Verification items for this drawing (mm, ordinates from the low corner). Give positions to 0.01 mm unless a question says otherwise; leave off trailing zeros. Loops run counter-clockwise (first coordinate to the right, second up) from the corner with the lowest first, then second, coordinate; pieces in that order, holes last. Notation, with made-up numbers: M 44.25,24.25 L 97.25,24.25 A31 ccw 97.25,54.25 Z; hole C 18.25,73.25 d8. An arc over 180 degrees is marked long. Use one line per item in the form item = value.
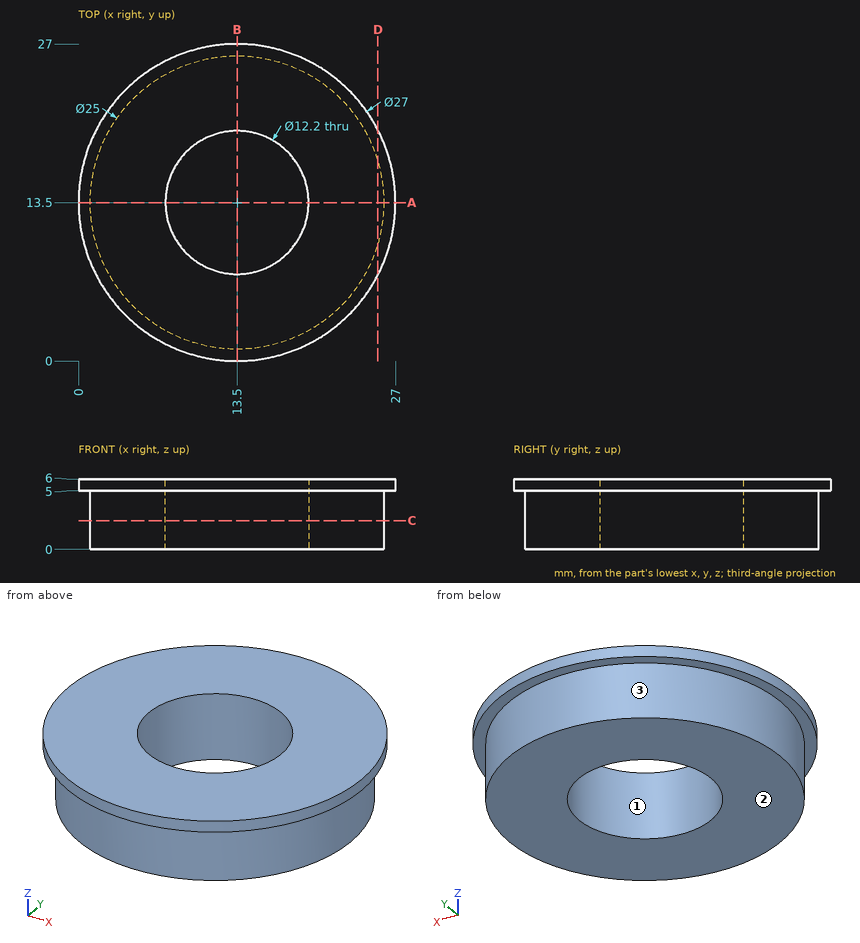
1) Depth check by flat-ended pin: pin 1 Ø1 at (x, z) = (17.5, 3.5) entering from -Y; pin 2 Ø4 at (x, y) = (20.5, 7) entering from -Z; pin 3 Ø1.5 at (x, z) = (21, 4) entering from -Y. Enter the tip coordinate at first touch or a pass-through.
Evaluation:
pin_1 = 1.5
pin_2 = 0
pin_3 = 2.98
2) Section check D-D (x = 25.5). Record the cut outline in (y, z), then the cut area to 3 significant figures.
Evaluation:
outline = M 7.32,5 L 10,5 L 10,0 L 17,0 L 17,5 L 19.68,5 L 19.68,6 L 7.32,6 Z
area = 47.4 mm^2
3) Section check C-C (z = 2.45). Record the cut outline in (x, y), then the cut area to 3 significant figures.
Evaluation:
outline = C 13.5,13.5 d25; hole C 13.5,13.5 d12.2
area = 374 mm^2
4) Section check A-A (y = 13.5). Record the cut outline in (x, z).
Evaluation:
outline = M 0,5 L 1,5 L 1,0 L 7.4,0 L 7.4,6 L 0,6 Z; M 19.6,0 L 26,0 L 26,5 L 27,5 L 27,6 L 19.6,6 Z
5) Release check for a two-part mould opening along X. For the marked faces 1, 2 and 3 record: pulls with the +X half, pulls with the -X half, needs draft (parallel to the pull), parting line crosses it, or undercut.
Evaluation:
face_1 = undercut
face_2 = needs draft
face_3 = parting line crosses it
6) Scan lines: line 1 (Y direction, x = 13.5, z = 4.1); line 2 (Z direction, x = 25.75, y = 9.5); line 3 (Y direction, x = 18.5, z = 3.9). Record each from-to range of solid material in increasing order.
Evaluation:
line_1 = 1 to 7.4, 19.6 to 26
line_2 = 5 to 6
line_3 = 2.04 to 10.01, 16.99 to 24.96
